from build123d import *

# Parameters (mm, degrees)
BOSS_EXTRUDE1_DEPTH = 67
SKETCH2_W           = 59.2
SKETCH2_H           = 17.698005222
CUT_EXTRUDE1_DEPTH  = 50.18617341
SKETCH3_W           = 2.5
SKETCH3_H           = 2.875
CUT_EXTRUDE2_DEPTH  = 81.40340279


with BuildPart() as part:
    # Sketch1 → Boss-Extrude1 (new body)
    with BuildSketch(Plane.XY):
        with BuildLine():
            Line((-13.748013557, 3.628954741), (-19.413054129, 4.660133913))
            Line((-19.413054129, 4.660133913), (-18.875806853, 7.611636134))
            Line((-18.875806853, 7.611636134), (-21.532158853, 8.095158683))
            Line((-21.532158853, 8.095158683), (-22.069406129, 5.143656461))
            Line((-22.069406129, 5.143656461), (-34.942701024, 7.48691833))
            Line((-34.942701024, 7.48691833), (-34.405453748, 10.438420552))
            Line((-34.405453748, 10.438420552), (-37.061805748, 10.9219431))
            Line((-37.061805748, 10.9219431), (-37.599053024, 7.970440879))
            Line((-37.599053024, 7.970440879), (-43.08617341, 8.969234123))
            Line((-43.08617341, 8.969234123), (-43.08617341, 0.15))
            Line((-43.08617341, 0.15), (9.1, 0.15))
            Line((9.1, 0.15), (9.1, 8.999002611))
            Line((9.1, 8.999002611), (-3.711145872, 8.999002611))
            ThreePointArc((-3.711145872, 8.999002611), (-7.792859586, 4.563205458), (-13.748013557, 3.628954741))
        make_face()
    extrude(amount=BOSS_EXTRUDE1_DEPTH)

    # Sketch2 → Cut-Extrude1 (cut)
    with BuildSketch(Plane.ZY.offset(43.08617341)):
        with Locations((33.5, 8.999002611)):
            Rectangle(SKETCH2_W, SKETCH2_H)
    extrude(amount=-CUT_EXTRUDE1_DEPTH, mode=Mode.SUBTRACT)

    # Sketch3 → Cut-Extrude2 (cut, through all)
    with BuildSketch(Plane(origin=(0, 0, 0), x_dir=(-1, 0, 0), z_dir=(0, 0, -1))):
        with Locations((29.25, 1.4375)):
            Rectangle(SKETCH3_W, SKETCH3_H)
    extrude(amount=-CUT_EXTRUDE2_DEPTH, mode=Mode.SUBTRACT)


solid = part.part
Verification items for the finished model (mm, model axes). A direction names the side the tool comes from. Round coordinates to 2 decimals unless told otherwise and drop trailing zeros. Loops run counter-clockwise (first coordinate to the right, second up) from the corner with the lowest first, then second, coordinate; pieces in that order, holes last. Notation, with made-up numbers: (88, -34.75) - (94, -34.75) arc R21 ccw to (94, -7.75) - close; hole circle Ø8 at (-34.5, 82.25). An arc over 180 degrees is marked (long way). Answer in a Markdown table with one row per item. Add a question column.
Q1. Section check D-D on z = 25. Enter the section's corners in (x, y), plus the area to 3 significant figures.
Q2. Release check for a two-part mould opening along X. For faces 4 (the face through (-16.541, 4.137, 65.023)), 5 (the face through (-35.715, 10.677, 65.023)), 6 (the face through (-18, 4, 63.1)) record: pulls with the +X half, pulls with the -X half, needs draft (parallel to the pull), parting line crosses it, or undercut.
Q3. Section check C-C on x = -23.5. Enter the section's corners in (y, z), plus the area to 3 significant figures.
Q4. Material ranges on line 1 (Z direction, x = -7, y = 1); line 2 (X direction, y = 5.25, z = 17.5), recorded low to high.
Q5. Section check B-B on y = 6. Enter the section's corners in (x, z), plus the area to 3 significant figures.
Q6. Gauge pin test, flat ends, axial feed: pin 1 (1 mm diameter, centred on x = -25.5, y = 2.5, fed in from -Z); pin 2 (1 mm diameter, centred on x = -15, y = 4.5, fed in from -Z); pin 3 (5 mm diameter, centred on y = 4.5, z = 28, fed in from -X). Record the tip position at first contact, or that the pin passes through.
Q7. Tool access check on faces 1 (the face through (-30.5, 1, 2)), 2 (the face through (-34.68, 8.94, 1.92)), 3 (the face through (-21.797, 6.64, 65.023)). Record the directions out of +Z, -Z, +X, -X, +Y, -Y that give a thin tool (end or side, any length) a straight path to the whole face; none if there is none.
Q8. Section check A-A on x = 1.5. Enter the section's corners in (y, z), plus the area to 3 significant figures.
Found:
| question | item | result |
|---|---|---|
| 1 | outline | (7.1, 0.15) - (9.1, 0.15) - (9.1, 9) - (7.1, 9) - close |
| 1 | area | 17.7 mm² |
| 2 | face 4 | undercut |
| 2 | face 5 | pulls with the +X half |
| 2 | face 6 | needs draft |
| 3 | outline | (0.15, 0) - (5.4, 0) - (5.4, 3.9) - (0.15, 3.9) - close; (0.15, 63.1) - (5.4, 63.1) - (5.4, 67) - (0.15, 67) - close |
| 3 | area | 41.0 mm² |
| 4 | line 1 | z = 0 to 3.9, 63.1 to 67 |
| 4 | line 2 | x = 7.1 to 9.1 |
| 5 | outline | (-43.09, 0) - (-26.77, 0) - (-26.77, 3.9) - (-43.09, 3.9) - close; (-43.09, 63.1) - (-26.77, 63.1) - (-26.77, 67) - (-43.09, 67) - close; (-21.91, 0) - (-19.17, 0) - (-19.17, 3.9) - (-21.91, 3.9) - close; (-21.91, 63.1) - (-19.17, 63.1) - (-19.17, 67) - (-21.91, 67) - close; (-5.8, 0) - (9.1, 0) - (9.1, 67) - (-5.8, 67) - (-5.8, 63.1) - (7.1, 63.1) - (7.1, 3.9) - (-5.8, 3.9) - close |
| 5 | area | 383 mm² |
| 6 | pin 1 | stops at z = 0 |
| 6 | pin 2 | passes through |
| 6 | pin 3 | stops at x = 7.1 |
| 7 | face 1 | +Z, -Z, -Y |
| 7 | face 2 | +Z, -Z |
| 7 | face 3 | +Z, -Z, +Y |
| 8 | outline | (0.15, 0) - (9, 0) - (9, 3.9) - (0.15, 3.9) - close; (0.15, 63.1) - (9, 63.1) - (9, 67) - (0.15, 67) - close |
| 8 | area | 69.0 mm² |
